from build123d import *

# Parameters (mm, degrees)
CYLINDER023_R                 = 2
CYLINDER023_DEPTH             = 10
CYLINDER024_R                 = 2
CYLINDER024_DEPTH             = 10
CYLINDER025_R                 = 2
CYLINDER025_DEPTH             = 10
CYLINDER020_R                 = 1.65
CYLINDER020_DEPTH             = 10
CYLINDER021_R                 = 1.65
CYLINDER021_DEPTH             = 10
CYLINDER022_R                 = 20.75
CYLINDER022_DEPTH             = 6
BOX005_W                      = 40
BOX005_H                      = 4.85
BOX005_DEPTH                  = 21
CHAMFER007_SIZE               = 2
CYLINDER019_R                 = 1.6
CYLINDER019_DEPTH             = 3
CYLINDER018_R                 = 1.6
CYLINDER018_DEPTH             = 3
CHAMFER006_SIZE               = 0.4
CYLINDER017_R                 = 20.9
CYLINDER017_DEPTH             = 6
BOX004_W                      = 40
BOX004_H                      = 13
BOX004_DEPTH                  = 5
CHAMFER008_SIZE               = 2
CHAMFER009_SIZE               = 0.4
CHAMFER009002_SIZE            = 0.4
CHAMFER009002_ROLL_ANGLE      = 180
CHAMFER009002_PLACEMENT_ANGLE = -90


with BuildPart() as cylinder023:
    # Cylinder023 → Cylinder023 (new body)
    with BuildSketch(Plane(origin=(0, -20, 11), x_dir=(1, 0, 0), z_dir=(0, -1, 0))):
        Circle(CYLINDER023_R)
    extrude(amount=CYLINDER023_DEPTH)


with BuildPart() as cylinder024:
    # Cylinder024 → Cylinder024 (new body)
    with BuildSketch(Plane(origin=(-8, -20, 11), x_dir=(1, 0, 0), z_dir=(0, -1, 0))):
        Circle(CYLINDER024_R)
    extrude(amount=CYLINDER024_DEPTH)


with BuildPart() as fusion001025:
    # Cylinder025 → Cylinder025 (new body)
    with BuildSketch(Plane(origin=(8, -20, 11), x_dir=(1, 0, 0), z_dir=(0, -1, 0))):
        Circle(CYLINDER025_R)
    extrude(amount=CYLINDER025_DEPTH)

    # Fusion001025: union Cylinder023, Cylinder024
    add(cylinder023.part)
    add(cylinder024.part)


with BuildPart() as cylinder020:
    # Cylinder020 → Cylinder020 (new body)
    with BuildSketch(Plane(origin=(16, -19, 17), x_dir=(1, 0, 0), z_dir=(0, -1, 0))):
        Circle(CYLINDER020_R)
    extrude(amount=CYLINDER020_DEPTH)


with BuildPart() as fusion001023:
    # Cylinder021 → Cylinder021 (new body)
    with BuildSketch(Plane(origin=(-16, -19, 17), x_dir=(1, 0, 0), z_dir=(0, -1, 0))):
        Circle(CYLINDER021_R)
    extrude(amount=CYLINDER021_DEPTH)

    # Fusion001023: union Cylinder020
    add(cylinder020.part)


with BuildPart() as cylinder022:
    # Cylinder022 → Cylinder022 (new body)
    with BuildSketch(Plane(origin=(0, -20, 36), x_dir=(1, 0, 0), z_dir=(0, -1, 0))):
        Circle(CYLINDER022_R)
    extrude(amount=CYLINDER022_DEPTH)


with BuildPart() as chamfer007:
    # Box005 → Box005 (new body)
    with BuildSketch(Plane(origin=(-20, -25, 0), x_dir=(1, 0, 0), z_dir=(0, 0, 1))):
        with Locations((20, 2.425)):
            Rectangle(BOX005_W, BOX005_H)
    extrude(amount=BOX005_DEPTH)

    # Cut004003006002: cut Cylinder022
    add(cylinder022.part, mode=Mode.SUBTRACT)

    # Cut004003006003: cut Fusion001023
    add(fusion001023.part, mode=Mode.SUBTRACT)

    # Chamfer007
    chamfer007_edges = [chamfer007.edges().sort_by_distance(p)[0] for p in [
        (-20, -22.575, 21),
        (20, -22.575, 21),
    ]]
    chamfer(chamfer007_edges, length=CHAMFER007_SIZE)


with BuildPart() as cylinder019:
    # Cylinder019 → Cylinder019 (new body)
    with BuildSketch(Plane(origin=(16, -16, 5), x_dir=(1, 0, 0), z_dir=(0, 0, 1))):
        Circle(CYLINDER019_R)
    extrude(amount=CYLINDER019_DEPTH)


with BuildPart() as chamfer006:
    # Cylinder018 → Cylinder018 (new body)
    with BuildSketch(Plane(origin=(-16, -16, 5), x_dir=(1, 0, 0), z_dir=(0, 0, 1))):
        Circle(CYLINDER018_R)
    extrude(amount=CYLINDER018_DEPTH)

    # Fusion001022: union Cylinder019
    add(cylinder019.part)

    # Chamfer006
    chamfer006_edges = [chamfer006.edges().sort_by_distance(p)[0] for p in [
        (-17.6, -16, 8),
        (14.4, -16, 8),
    ]]
    chamfer(chamfer006_edges, length=CHAMFER006_SIZE)


with BuildPart() as cylinder017:
    # Cylinder017 → Cylinder017 (new body)
    with BuildSketch(Plane.XY):
        Circle(CYLINDER017_R)
    extrude(amount=CYLINDER017_DEPTH)


with BuildPart() as chamfer009002:
    # Box004 → Box004 (new body)
    with BuildSketch(Plane(origin=(-20, -25, 0), x_dir=(1, 0, 0), z_dir=(0, 0, 1))):
        with Locations((20, 6.5)):
            Rectangle(BOX004_W, BOX004_H)
    extrude(amount=BOX004_DEPTH)

    # Chamfer008
    chamfer008_edges = [chamfer009002.edges().sort_by_distance(p)[0] for p in [
        (-20, -12, 2.5),
        (20, -12, 2.5),
    ]]
    chamfer(chamfer008_edges, length=CHAMFER008_SIZE)

    # Cut004003006004: cut Cylinder017
    add(cylinder017.part, mode=Mode.SUBTRACT)

    # Fusion001024: union Chamfer007, Chamfer006
    add(chamfer007.part)
    add(chamfer006.part)

    # Cut004003006005: cut Fusion001025
    add(fusion001025.part, mode=Mode.SUBTRACT)

    # Chamfer009
    chamfer009_edges = [chamfer009002.edges().sort_by_distance(p)[0] for p in [
        (-10, -20.15, 11),
        (-2, -20.15, 11),
        (6, -20.15, 11),
    ]]
    chamfer(chamfer009_edges, length=CHAMFER009_SIZE)

    # Chamfer009002
    chamfer009002_edges = [chamfer009002.edges().sort_by_distance(p)[0] for p in [
        (19, -25, 20),
        (16.168725, -25, 21),
        (0, -25, 15.25),
        (-16.168725, -25, 21),
        (-19, -25, 20),
        (-17.65, -25, 17),
        (14.35, -25, 17),
        (-10, -25, 11),
        (-2, -25, 11),
        (6, -25, 11),
        (20, -25, 9.5),
        (0, -25, 0),
        (-20, -25, 9.5),
    ]]
    chamfer(chamfer009002_edges, length=CHAMFER009002_SIZE)


with BuildPart() as chamfer009002_1:
    # Chamfer009002 roll: moved
    add(chamfer009002.part.rotate(Axis((0, 0, 0), (1, 0, 0)), CHAMFER009002_ROLL_ANGLE))


with BuildPart() as chamfer009002_2:
    # Chamfer009002 placement: moved
    add(chamfer009002_1.part.moved(Location((0, 0, 50))).rotate(Axis((0, 0, 50), (0, 0, 1)), CHAMFER009002_PLACEMENT_ANGLE))


solid = chamfer009002_2.part
Here's how the part is built. I have some questions about the finished solid (model axes, mm). A direction names the side the tool comes from. Coordinates: 2 decimals unless noted, no trailing zeros. Write each loop counter-clockwise with the first axis right and the second up, starting at its lowest first coordinate (ties: lowest second). Pieces come first, ordered by that corner, then holes.
Item 1: I want a section at A-A on y = 0. Write out the boundary of the cut face in (x, z).
Item 2: Will these pins go through, and if not, where does the flat tip stop? pin 1 (6.5 mm diameter, centred on x = 15.5, y = -11, fed in from -Z); pin 2 (6.5 mm diameter, centred on y = -8, z = 39, fed in from -X); pin 3 (0.7 mm diameter, centred on x = 15.5, y = -15.5, fed in from -Z).
Item 3: On a 3-axis mill with a long thin cutter (end or side, diameter ignored), from which of +Z, -Z, +X, -X, +Y, -Y can I reach the whole of each face in a straight line? I mean faces 1 (the flat face through (24.803, -18.871, 30.157)), 2 (the cylindrical face through (14.92, -14.82, 43.72)). Say none if no direction works.
Item 4: If I drill on line 1 (Y direction, x = 22.25, z = 39); line 2 (Y direction, x = 22, z = 40.5); line 3 (Z direction, x = 23, y = 0), over which ranges is the centre line in solid material (lowest first)?
Item 5: If we mould it in two halves opening along Y, with no side actions, what happens to faces 3 (the cylindrical face through (23, -8, 41)), 4 (the cylindrical face through (22.34, -16.89, 31.61)), 5 (the flat face through (24.803, 18.871, 30.157)), 6 (the flat face through (12, 17.6, 47.5))? For each: +Y half, -Y half, draft (parallel to the pull), parting line (faces both ways), or undercut.
Item 6: I want a section at D-D on x = 19.5. Write out the boundary of the cut face in (y, z).
Item 7: I want a section at C-C on x = 22. Write out the boundary of the cut face in (y, z).
Item 8: I want a section at B-B on z = 44. Write out the boundary of the cut face in (x, y).
Findings below:
1. outline: (20.15, 34.75) - (24.6, 34.75) - (25, 35.15) - (25, 36.6) - (24.6, 37) - (20.55, 37) - (20.15, 36.6) - close; (20.15, 41.4) - (20.55, 41) - (24.6, 41) - (25, 41.4) - (25, 49.6) - (24.6, 50) - (20.15, 50) - close
2. pin 1: stops at z = 45
2. pin 2: stops at x = 20.15
2. pin 3: stops at z = 42
3. face 1: -Z, +X, -Y
3. face 2: -Z
4. line 1: y = -20 to -10, -6 to -2, 2 to 6, 10 to 20
4. line 2: y = -20 to -9.32, -6.68 to -1.32, 1.32 to 6.68, 9.32 to 20
4. line 3: z = 34.75 to 37, 41 to 50
5. face 3: undercut
5. face 4: undercut
5. face 5: +Y half
5. face 6: draft
6. outline: (-20, 45) - (-7.52, 45) - (-7.52, 50) - (-20, 50) - close; (7.52, 45) - (20, 45) - (20, 50) - (7.52, 50) - close
7. outline: (-20, 31) - (-18, 29) - (-14.34, 29) arc R20.75 cw to (14.34, 29) - (18, 29) - (20, 31) - (20, 50) - (-20, 50) - close; hole circle Ø3.3 at (-16, 33); hole circle Ø4 at (-8, 39); hole circle Ø4 at (0, 39); hole circle Ø4 at (8, 39); hole circle Ø3.3 at (16, 33)
8. outline: circle Ø3.2 at (16, -16); circle Ø3.2 at (16, 16); (20.15, -20) - (24.6, -20) - (25, -19.6) - (25, 19.6) - (24.6, 20) - (20.15, 20) - close
